```python
from build123d import *

# Parameters (mm, degrees)
SKETCH1_R           = 1.75
BOSS_EXTRUDE1_DEPTH = 2


with BuildPart() as part:
    # Sketch1 → Boss-Extrude1 (new body)
    with BuildSketch(Plane.XY):
        with BuildLine():
            Line((0, 0), (0, 3.327095189))
            Line((0, 3.327095189), (7.929895835, 25.403579408))
            ThreePointArc((7.929895835, 25.403579408), (13.70124174, 31.117370669), (14.517783542, 23.037203368))
            Line((14.517783542, 23.037203368), (12.831302958, 18.342114962))
            ThreePointArc((12.831302958, 18.342114962), (12.721539225, 17.487494723), (12.981505781, 16.666007522))
            Line((12.981505781, 16.666007522), (19.598076211, 5.205771366))
            ThreePointArc((19.598076211, 5.205771366), (19.897777479, 4.482228501), (20, 3.705771366))
            Line((20, 3.705771366), (20, 0))
            Line((20, 0), (15, 0))
            Line((15, 0), (15, 2))
            Line((15, 2), (12.5, 2))
            Line((12.5, 2), (12.5, 3.098076211))
            ThreePointArc((12.5, 3.098076211), (12.448888739, 3.486304779), (12.299038106, 3.848076211))
            Line((12.299038106, 3.848076211), (9.848953011, 8.091748078))
            ThreePointArc((9.848953011, 8.091748078), (9.46684029, 8.290151551), (9.126092124, 8.026969566))
            Line((9.126092124, 8.026969566), (7.588309777, 3.745850569))
            ThreePointArc((7.588309777, 3.745850569), (7.522242352, 3.49612642), (7.5, 3.238769989))
            Line((7.5, 3.238769989), (7.5, 2))
            Line((7.5, 2), (5, 2))
            Line((5, 2), (5, 0))
            Line((5, 0), (0, 0))
        make_face()
        with Locations((12.18, 26.8823)):
            Circle(SKETCH1_R, mode=Mode.SUBTRACT)
    extrude(amount=BOSS_EXTRUDE1_DEPTH)


solid = part.part
```
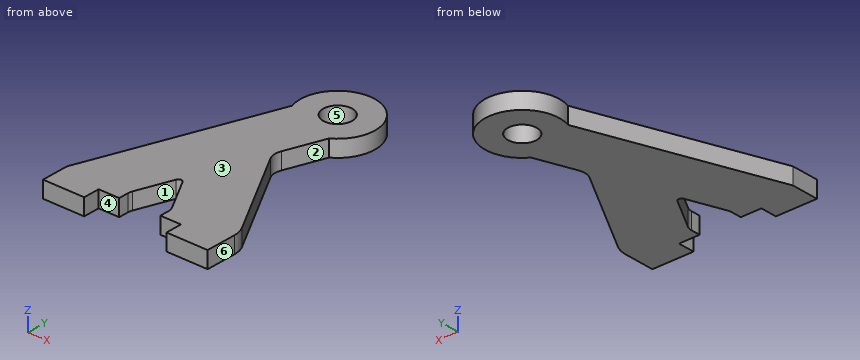
Check sheet for the modelled part. Datum: model origin and axes. Units: mm. Face numbers are marked on the shaded views. A direction names the side the tool comes from. Give positions to 0.01 mm unless a question says otherwise; leave off trailing zeros. Order: outer loops, then holes, each group sorted by start corner. A loop starts at its lowest first (then second) coordinate and runs counter-clockwise, first axis right, second up. Notation, with made-up numbers: M 44,-7.5 L 100,-7.5 A24 ccw 100,14.5 Z; hole C 13.25,0 d3. An arc over 180 degrees is marked long. Answer in a Markdown table with one row per item.
1) Cross-section at C-C, the plane y = 29.5. Enter the section's corners in (x, z).
Filled sheet:
| item | result |
|---|---|
| outline | M 8.52,0 L 15.84,0 L 15.84,2 L 8.52,2 Z |
2) Thickness scan on L1, parallel to X at y = 1.5, z = 1.4; L2, parallel to X at y = 27, z = 0.3; L3, parallel to Y at x = 15.75, z = 1.5. Record the ranges inside material, lowest first. Write a range as [from, to].
Filled sheet:
| item | result |
|---|---|
| L1 | x = [0, 5], [15, 20] |
| L2 | x = [7.68, 10.43], [13.93, 16.68] |
| L3 | y = [0, 11.87], [24.14, 29.62] |
3) Release check for a two-part mould opening along Y. For the marked faces 4, 5 and 6 record: +Y half, -Y half, draft (parallel to the pull), parting line (faces both ways), or undercut.
Filled sheet:
| item | result |
|---|---|
| face 4 | -Y half |
| face 5 | undercut |
| face 6 | draft |
4) Cross-section at A-A, the plane z = 0.35. Enter the section's corners in (x, y), plus the area to 3 significant figures.
Filled sheet:
| item | result |
|---|---|
| outline | M 0,0 L 5,0 L 5,2 L 7.5,2 L 7.5,3.24 A1.5 cw 7.59,3.75 L 9.13,8.03 A0.4 cw 9.85,8.09 L 12.3,3.85 A1.5 cw 12.5,3.1 L 12.5,2 L 15,2 L 15,0 L 20,0 L 20,3.71 A3 ccw 19.6,5.21 L 12.98,16.67 A2 cw 12.83,18.34 L 14.52,23.04 A4.5 ccw long 7.93,25.4 L 0,3.33 Z; hole C 12.18,26.88 d3.5 |
| area | 320 mm2 |
5) Access from +Z, -Z, +X, -X, +Y, -Y to the whole of each face (thin tool, end or side, straight path). Record for the marked faces 1, 2 and 3.
Filled sheet:
| item | result |
|---|---|
| face 1 | +Z, -Z, -Y |
| face 2 | +Z, -Z, +X |
| face 3 | +Z, +X, -X, +Y, -Y |
6) Cross-section at B-B, the plane x = 17.25. Enter the section's corners in (y, z), plus the area to 3 significant figures.
Filled sheet:
| item | result |
|---|---|
| outline | M 0,0 L 9.27,0 L 9.27,2 L 0,2 Z |
| area | 18.5 mm2 |
